```python
from build123d import *

# Parameters (mm, degrees)
SKETCH1_R           = 25.4
BOSS_EXTRUDE1_DEPTH = 1.5
BOSS_EXTRUDE2_START = 1.5
SKETCH1_3_R         = 20.066
SKETCH1_3_R_2       = 18.415
BOSS_EXTRUDE2_DEPTH = 4
BOSS_EXTRUDE3_START = 5.5
SKETCH1_4_R         = 25.4
SKETCH1_4_R_2       = 20.066
SKETCH1_4_R_3       = 18.415
BOSS_EXTRUDE3_DEPTH = 1.5
BOSS_EXTRUDE4_START = 7
SKETCH1_5_R         = 20.066
SKETCH1_5_R_2       = 18.415
BOSS_EXTRUDE4_DEPTH = 4
BOSS_EXTRUDE5_START = 11
SKETCH1_6_R         = 25.4
SKETCH1_6_R_2       = 20.066
SKETCH1_6_R_3       = 18.415
BOSS_EXTRUDE5_DEPTH = 1.5
BOSS_EXTRUDE6_START = 1.5
SKETCH1_7_R         = 5
BOSS_EXTRUDE6_DEPTH = 5


with BuildPart() as part:
    # Sketch1 → Boss-Extrude1 (new body)
    with BuildSketch(Plane(origin=(0, 0, 0), x_dir=(1, 0, 0), z_dir=(0, 1, 0))):
        with Locations(Location((0, 0, 0), (0, 0, 270))):
            Circle(SKETCH1_R)
    extrude(amount=BOSS_EXTRUDE1_DEPTH)

    # Sketch1<3> → Boss-Extrude2 (add)
    with BuildSketch(Plane(origin=(0, 0, 0), x_dir=(1, 0, 0), z_dir=(0, 1, 0)).offset(BOSS_EXTRUDE2_START)):
        with Locations(Location((0, 0, 0), (0, 0, 270))):
            Circle(SKETCH1_3_R)
        with Locations(Location((0, 0, 0), (0, 0, 270))):
            Circle(SKETCH1_3_R_2, mode=Mode.SUBTRACT)
    extrude(amount=BOSS_EXTRUDE2_DEPTH)

    # Sketch1<4> → Boss-Extrude3 (add)
    # profile 1 of 2: a face of its own
    with BuildSketch(Plane(origin=(0, 0, 0), x_dir=(1, 0, 0), z_dir=(0, 1, 0)).offset(BOSS_EXTRUDE3_START)):
        with Locations(Location((0, 0, 0), (0, 0, 270))):
            Circle(SKETCH1_4_R)
        with Locations(Location((0, 0, 0), (0, 0, 270))):
            Circle(SKETCH1_4_R_2, mode=Mode.SUBTRACT)
    # profile 2 of 2: a face of its own
    with BuildSketch(Plane(origin=(0, 0, 0), x_dir=(1, 0, 0), z_dir=(0, 1, 0)).offset(BOSS_EXTRUDE3_START)):
        with Locations(Location((0, 0, 0), (0, 0, 270))):
            Circle(SKETCH1_4_R_2)
        with Locations(Location((0, 0, 0), (0, 0, 270))):
            Circle(SKETCH1_4_R_3, mode=Mode.SUBTRACT)
    extrude(amount=BOSS_EXTRUDE3_DEPTH)

    # Sketch1<5> → Boss-Extrude4 (add)
    with BuildSketch(Plane(origin=(0, 0, 0), x_dir=(1, 0, 0), z_dir=(0, 1, 0)).offset(BOSS_EXTRUDE4_START)):
        with Locations(Location((0, 0, 0), (0, 0, 270))):
            Circle(SKETCH1_5_R)
        with Locations(Location((0, 0, 0), (0, 0, 270))):
            Circle(SKETCH1_5_R_2, mode=Mode.SUBTRACT)
    extrude(amount=BOSS_EXTRUDE4_DEPTH)

    # Sketch1<6> → Boss-Extrude5 (add)
    # profile 1 of 2: a face of its own
    with BuildSketch(Plane(origin=(0, 0, 0), x_dir=(1, 0, 0), z_dir=(0, 1, 0)).offset(BOSS_EXTRUDE5_START)):
        with Locations(Location((0, 0, 0), (0, 0, 270))):
            Circle(SKETCH1_6_R)
        with Locations(Location((0, 0, 0), (0, 0, 270))):
            Circle(SKETCH1_6_R_2, mode=Mode.SUBTRACT)
    # profile 2 of 2: a face of its own
    with BuildSketch(Plane(origin=(0, 0, 0), x_dir=(1, 0, 0), z_dir=(0, 1, 0)).offset(BOSS_EXTRUDE5_START)):
        with Locations(Location((0, 0, 0), (0, 0, 270))):
            Circle(SKETCH1_6_R_2)
        with Locations(Location((0, 0, 0), (0, 0, 270))):
            Circle(SKETCH1_6_R_3, mode=Mode.SUBTRACT)
    extrude(amount=BOSS_EXTRUDE5_DEPTH)

    # Sketch1<7> → Boss-Extrude6 (add)
    with BuildSketch(Plane(origin=(0, 0, 0), x_dir=(1, 0, 0), z_dir=(0, 1, 0)).offset(BOSS_EXTRUDE6_START)):
        with Locations(Location((0, 0, 0), (0, 0, 270))):
            Circle(SKETCH1_7_R)
    extrude(amount=BOSS_EXTRUDE6_DEPTH)


solid = part.part
```
Here's how the part is built. I have some questions about the finished solid (model axes, mm). A direction names the side the tool comes from. Coordinates: 2 decimals unless noted, no trailing zeros. Order: outer loops, then holes, each group sorted by start corner. A loop starts at its lowest first (then second) coordinate and runs counter-clockwise, first axis right, second up. Notation, with made-up numbers: (14.5, -14) - (27.5, -14) arc R19 cw to (27.5, -8) - close; hole circle Ø10 at (1.25, 21). An arc over 180 degrees is marked (long way). One line per question, with ' | ' between items.
(1) Suppose I cut it at B-B on z = 0. List the corners of the cut face in (x, y) for me (3 decimals).
Report:
outline: (-25.4, 0) - (25.4, 0) - (25.4, 1.5) - (20.066, 1.5) - (20.066, 5.5) - (25.4, 5.5) - (25.4, 7) - (20.066, 7) - (20.066, 11) - (25.4, 11) - (25.4, 12.5) - (18.415, 12.5) - (18.415, 1.5) - (5, 1.5) - (5, 6.5) - (-5, 6.5) - (-5, 1.5) - (-18.415, 1.5) - (-18.415, 12.5) - (-25.4, 12.5) - (-25.4, 11) - (-20.066, 11) - (-20.066, 7) - (-25.4, 7) - (-25.4, 5.5) - (-20.066, 5.5) - (-20.066, 1.5) - (-25.4, 1.5) - close
(2) Suppose I cut it at D-D on y = 10. List the corners of the cut face in (x, z) for me (3 decimals).
Report:
outline: circle Ø40.132 at (0, 0); hole circle Ø36.83 at (0, 0)
(3) If we mould it in two halves opening along X, with no side actions, what happens to faces 1 (the flat face through (0, 6.5, 0)), 2 (the cylindrical face through (-19.6, 3.5, -4.3)), 3 (the flat face through (8, 12.5, 17)), 4 (the cylindrical face through (-11.21, 6.92, -14.61))? For each: pulls with the +X half, pulls with the -X half, needs draft (parallel to the pull), parting line crosses it, or undercut.
Report:
face 1: undercut | face 2: parting line crosses it | face 3: needs draft | face 4: undercut
(4) Suppose I cut it at A-A on y = 3. List the corners of the cut face in (x, z) for me (3 decimals), and give its area (3 significant figures).
Report:
outline: circle Ø40.132 at (0, 0); circle Ø10 at (0, 0); hole circle Ø36.83 at (0, 0) | area: 278 mm2
(5) Suppose I cut it at C-C on x = 0. List the corners of the cut face in (y, z) for me (3 decimals), and give its area (3 significant figures).
Report:
outline: (0, -25.4) - (1.5, -25.4) - (1.5, -20.066) - (5.5, -20.066) - (5.5, -25.4) - (7, -25.4) - (7, -20.066) - (11, -20.066) - (11, -25.4) - (12.5, -25.4) - (12.5, -18.415) - (1.5, -18.415) - (1.5, -5) - (6.5, -5) - (6.5, 5) - (1.5, 5) - (1.5, 18.415) - (12.5, 18.415) - (12.5, 25.4) - (11, 25.4) - (11, 20.066) - (7, 20.066) - (7, 25.4) - (5.5, 25.4) - (5.5, 20.066) - (1.5, 20.066) - (1.5, 25.4) - (0, 25.4) - close | area: 195 mm2
(6) Will these pins go through, and if not, where does the flat tip stop? pin 1 (1.5 mm diameter, centred on x = 12.5, y = 3, fed in from -Z); pin 2 (3 mm diameter, centred on x = -9.5, z = -10, fed in from +Y); pin 3 (5 mm diameter, centred on y = 4, z = 8.5, fed in from -X); pin 4 (8 mm diameter, centred on x = 18, z = -20, fed in from +Y).
Report:
pin 1: stops at z = -16.27 | pin 2: stops at y = 1.5 | pin 3: stops at x = -24.55 | pin 4: stops at y = 12.5
(7) For faces 5 (the flat face through (8, 11, 19)), 6 (the cylindrical face through (-4.88, 3.96, -1.08)), 7 (the flat face through (0, 0, 0)), which set-ups out of +Z, -Z, +X, -X, +Y, -Y let a thin tool reach every point of the face, with its end or its side?
Report:
face 5: none | face 6: +Y | face 7: +Z, -Z, +X, -X, -Y
(8) If I drill on L1, parallel to Y at x = 15.5, z = -14; L2, parallel to X at y = 4.75, z = 0 (3 decimals); L3, parallel to X at y = 3, z = 3, over which ranges is the centre line in solid material (lowest first)?
Report:
L1: y = 0 to 1.5, 5.5 to 7, 11 to 12.5 | L2: x = -20.066 to -18.415, -5 to 5, 18.415 to 20.066 | L3: x = -19.84 to -18.17, -4 to 4, 18.17 to 19.84
